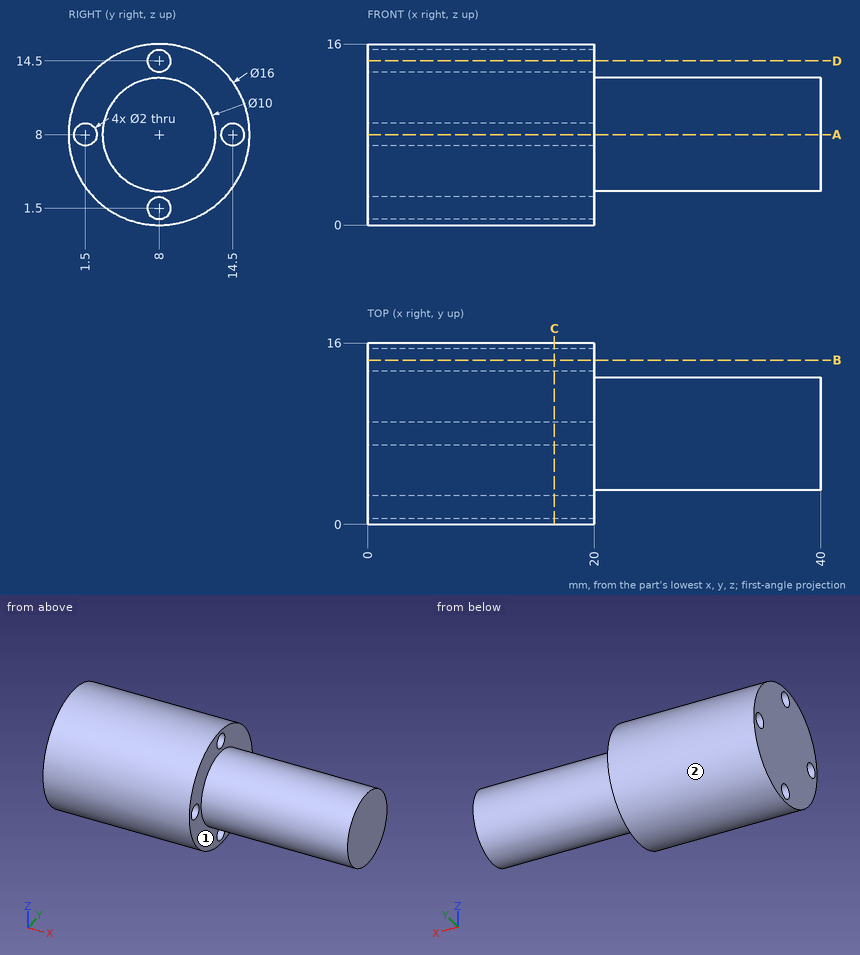
Answer from the drawing. Dimensions are ordinates in mm from the lowest x, y and z of the part. A direction names the side the tool comes from. Coordinates: 2 decimals unless noted, no trailing zeros. Loops run counter-clockwise (first coordinate to the right, second up) from the corner with the lowest first, then second, coordinate; pieces in that order, holes last. Notation, with made-up numbers: (71.5, 25.5) -> (127.5, 25.5) arc R35 ccw to (127.5, 57.5) -> close; hole circle Ø3 at (-12, 1). An arc over 180 degrees is marked (long way). Answer as CSV lines item,"result".
Q1. The part is cut by section A-A on z = 8. Write down the section's boundary in (x, y), and give its area (3 significant figures).
Findings:
outline,"(0, 0) -> (20, 0) -> (20, 0.5) -> (0, 0.5) -> close; (0, 2.5) -> (20, 2.5) -> (20, 3) -> (40, 3) -> (40, 13) -> (20, 13) -> (20, 13.5) -> (0, 13.5) -> close; (0, 15.5) -> (20, 15.5) -> (20, 16) -> (0, 16) -> close"
area,"440 mm²"
Q2. Each of these flat-tipped pins is pushed along its axis until it touches: pin 1 (1.5 mm diameter, centred on x = 29.5, z = 2, fed in from -Y); pin 2 (1 mm diameter, centred on x = 24.5, y = 12, fed in from +Z); pin 3 (8 mm diameter, centred on x = 31, z = 10, fed in from +Y); pin 4 (2.5 mm diameter, centred on y = 8, z = 1.5, fed in from +X). Where does it stop, or does it pass through?
Findings:
pin 1,"passes through"
pin 2,"stops at z = 11.57"
pin 3,"stops at y = 13"
pin 4,"stops at x = 20"
Q3. The part is cut by section B-B on y = 14.5. Write down the section's boundary in (x, z), and give its area (3 significant figures).
Findings:
outline,"(0, 3.34) -> (20, 3.34) -> (20, 7) -> (0, 7) -> close; (0, 9) -> (20, 9) -> (20, 12.66) -> (0, 12.66) -> close"
area,"147 mm²"
Q4. A tool of negligible diameter and unlimited length cuts with its end or side. For the marked faces 1 and 2, from which of +Z, -Z, +X, -X, +Y, -Y can it reach the whole face along a straight path? Write none if from no direction.
Findings:
face 1,"+X"
face 2,"+X, -X"
Q5. Find the intervals of material crossed by probe 1 along X at (y, z) = (6, 2); probe 2 along Z at (x, y) = (32, 8.25); probe 3 along Z at (x, y) = (10, 14.5), in increasing order.
Findings:
probe 1,"x = 0 to 20"
probe 2,"z = 3.01 to 12.99"
probe 3,"z = 3.34 to 7, 9 to 12.66"
Q6. The part is cut by section C-C on x = 16.5. Write down the section's boundary in (y, z).
Findings:
outline,"circle Ø16 at (8, 8); hole circle Ø2 at (1.5, 8); hole circle Ø2 at (8, 1.5); hole circle Ø2 at (8, 14.5); hole circle Ø2 at (14.5, 8)"
